from build123d import *

# Parameters (mm, degrees)
COMPACT_HORN_CENTER_OD6P9_PROFILE_R        = 3.45
COMPACT_HORN_CENTER_OD6P9_DEPTH            = 1.5
HORIZONTAL_BLADES_ASSUMED_WIDTH4_PROFILE_W = 16.3
HORIZONTAL_BLADES_ASSUMED_WIDTH4_PROFILE_H = 4
HORIZONTAL_BLADES_ASSUMED_WIDTH4_DEPTH     = 1.5
VERTICAL_BLADES_ASSUMED_WIDTH4_PROFILE_W   = 4
VERTICAL_BLADES_ASSUMED_WIDTH4_PROFILE_H   = 16.3
VERTICAL_BLADES_ASSUMED_WIDTH4_DEPTH       = 1.5
ROUNDED_BLADE_TIPS_R                       = 2
ROUNDED_TIPS_SPAN20P3_DEPTH                = 1.5
HUB_TOTAL_HEIGHT2P5_START                  = -1
HUB_TOTAL_HEIGHT2P5_PROFILE_R              = 3.45
HUB_TOTAL_HEIGHT2P5_DEPTH                  = 1
PURCHASED_SPLINE_INTERNALS_OMITTED_START   = -50
PURCHASED_SPLINE_INTERNALS_OMITTED_PROFI_R = 2.55
PURCHASED_SPLINE_INTERNALS_OMITTED_DEPTH   = 65.432428763
UNMODIFIED_STOCK_PILOT_HOLES_START         = -50
UNMODIFIED_STOCK_PILOT_HOLES_PROFILE_R     = 0.5
UNMODIFIED_STOCK_PILOT_HOLES_DEPTH         = 65.432428763


with BuildPart() as part:
    # Compact_horn_center_OD6p9_profile → Compact_horn_center_OD6p9 (new body)
    with BuildSketch(Plane.XY):
        Circle(COMPACT_HORN_CENTER_OD6P9_PROFILE_R)
    extrude(amount=COMPACT_HORN_CENTER_OD6P9_DEPTH)

    # Horizontal_blades_assumed_width4_profile → Horizontal_blades_assumed_width4 (add)
    with BuildSketch(Plane.XY):
        Rectangle(HORIZONTAL_BLADES_ASSUMED_WIDTH4_PROFILE_W, HORIZONTAL_BLADES_ASSUMED_WIDTH4_PROFILE_H)
    extrude(amount=HORIZONTAL_BLADES_ASSUMED_WIDTH4_DEPTH)

    # Vertical_blades_assumed_width4_profile → Vertical_blades_assumed_width4 (add)
    with BuildSketch(Plane.XY):
        Rectangle(VERTICAL_BLADES_ASSUMED_WIDTH4_PROFILE_W, VERTICAL_BLADES_ASSUMED_WIDTH4_PROFILE_H)
    extrude(amount=VERTICAL_BLADES_ASSUMED_WIDTH4_DEPTH)

    # Rounded_blade_tips → Rounded_tips_span20p3 (add)
    with BuildSketch(Plane.XY):
        with Locations((8.15, 0)):
            Circle(ROUNDED_BLADE_TIPS_R)
        with Locations((-8.15, 0)):
            Circle(ROUNDED_BLADE_TIPS_R)
        with Locations((0, 8.15)):
            Circle(ROUNDED_BLADE_TIPS_R)
        with Locations((0, -8.15)):
            Circle(ROUNDED_BLADE_TIPS_R)
    extrude(amount=ROUNDED_TIPS_SPAN20P3_DEPTH)

    # Hub_total_height2p5_profile → Hub_total_height2p5 (add)
    with BuildSketch(Plane.XY.offset(HUB_TOTAL_HEIGHT2P5_START)):
        with Locations(Location((0, 0, 0), (0, 0, 215.43015836))):
            Circle(HUB_TOTAL_HEIGHT2P5_PROFILE_R)
    extrude(amount=HUB_TOTAL_HEIGHT2P5_DEPTH)

    # Purchased_spline_internals_omitted_profile → Purchased_spline_internals_omitted (cut, through all)
    with BuildSketch(Plane.XY.offset(PURCHASED_SPLINE_INTERNALS_OMITTED_START)):
        Circle(PURCHASED_SPLINE_INTERNALS_OMITTED_PROFI_R)
    extrude(amount=PURCHASED_SPLINE_INTERNALS_OMITTED_DEPTH, mode=Mode.SUBTRACT)

    # Unmodified_stock_pilot_holes_profile → Unmodified_stock_pilot_holes (cut, through all)
    with BuildSketch(Plane.XY.offset(UNMODIFIED_STOCK_PILOT_HOLES_START)):
        with Locations((-8.3, 0)):
            Circle(UNMODIFIED_STOCK_PILOT_HOLES_PROFILE_R)
        with Locations((-6.3, 0)):
            Circle(UNMODIFIED_STOCK_PILOT_HOLES_PROFILE_R)
        with Locations((-4.3, 0)):
            Circle(UNMODIFIED_STOCK_PILOT_HOLES_PROFILE_R)
        with Locations((4.3, 0)):
            Circle(UNMODIFIED_STOCK_PILOT_HOLES_PROFILE_R)
        with Locations((6.3, 0)):
            Circle(UNMODIFIED_STOCK_PILOT_HOLES_PROFILE_R)
        with Locations((8.3, 0)):
            Circle(UNMODIFIED_STOCK_PILOT_HOLES_PROFILE_R)
        with Locations((0, -8.3)):
            Circle(UNMODIFIED_STOCK_PILOT_HOLES_PROFILE_R)
        with Locations((0, -6.3)):
            Circle(UNMODIFIED_STOCK_PILOT_HOLES_PROFILE_R)
        with Locations((0, -4.3)):
            Circle(UNMODIFIED_STOCK_PILOT_HOLES_PROFILE_R)
        with Locations((0, 4.3)):
            Circle(UNMODIFIED_STOCK_PILOT_HOLES_PROFILE_R)
        with Locations((0, 6.3)):
            Circle(UNMODIFIED_STOCK_PILOT_HOLES_PROFILE_R)
        with Locations((0, 8.3)):
            Circle(UNMODIFIED_STOCK_PILOT_HOLES_PROFILE_R)
    extrude(amount=UNMODIFIED_STOCK_PILOT_HOLES_DEPTH, mode=Mode.SUBTRACT)


solid = part.part
Input: part model. Units: mm. Frame: model coordinates. A direction names the side the tool comes from. Round coordinates to 2 decimals unless told otherwise and drop trailing zeros. Order: outer loops, then holes, each group sorted by start corner. A loop starts at its lowest first (then second) coordinate and runs counter-clockwise, first axis right, second up. Notation, with made-up numbers: (5.25, 48.25) - (29.25, 48.25) arc R23 ccw to (29.25, 83.25) - close; hole circle Ø3 at (3.25, -27). An arc over 180 degrees is marked (long way). Answer as a JSON object with one key per item and string values. Group by question number.
(1) Pin query (flat end, axial travel): P1, Ø2, axis at x = -6, y = 0.5, coming from the -Z side; P2, Ø1.2, axis at y = -6.5, z = 1, coming from the +X side; P3, Ø0.8, axis at x = 6, z = 0.5, coming from the -Y side. Return the tip coordinate at first contact, or that it passes through.
(2) Draft query along Y for faces 1 (the face through (-0.108, 3.812, 0.739)), 2 (the face through (-0.065, -5.804, 0.739)), 3 (the face through (2, -6, 1)), 4 (the face through (5, 2, 1)). Return one class per face: released by +Y, released by -Y, zero draft, split by the parting line, or undercut.
(3) Cut plane C-C (z = 0.8). Count the separate pieces of the cut face and the enclosed holes in it, then the cut area to 3 significant figures.
(4) Material intervals for probe 1 along Y at (x, z) = (8.3, 0.8); probe 2 along X at (y, z) = (-4.3, 0.6); probe 3 along X at (y, z) = (-3.75, 0.3), sorted ascending. Write a range as from..to.
(5) Reachability of faces 5 (the face through (-2, 2, 1.5)), 6 (the face through (2, 5, 1)), 7 (the face through (-6.8, 0, 0.7)), 8 (the face through (-2, 5, 1)), 9 (the face through (-2, -6, 1)) from +Z, -Z, +X, -X, +Y, -Y: full face, straight path, thin tool, end or side. Return the list, or none.
(6) Cut plane A-A (x = -4.3). Return loops of the section in (y, z), then the cut area to 3 significant figures.
(7) Cut plane D-D (z = -0.55). Return loops of the section in (x, y).
Here are the results:
{
 "1": {"P1": "stops at z = 0", "P2": "stops at x = 2", "P3": "stops at y = -2"},
 "2": {"face 1": "undercut", "face 2": "undercut", "face 3": "zero draft", "face 4": "released by +Y"},
 "3": {"separate pieces": "1", "enclosed holes": "13", "area": "111 mm^2"},
 "4": {"probe 1": "y = -1.99..-0.5, 0.5..1.99", "probe 2": "x = -2..-0.5, 0.5..2", "probe 3": "x = -2..2"},
 "5": {"face 5": "+Z, +X, -X, +Y, -Y", "face 6": "+Z, -Z, +X, +Y", "face 7": "+Z, -Z", "face 8": "+Z, -Z, -X, +Y", "face 9": "+Z, -Z, -X, -Y"},
 "6": {"outline": "(-2, 0) - (-0.5, 0) - (-0.5, 1.5) - (-2, 1.5) - close; (0.5, 0) - (2, 0) - (2, 1.5) - (0.5, 1.5) - close", "area": "4.50 mm^2"},
 "7": {"outline": "circle Ø6.9 at (0, 0); hole circle Ø5.1 at (0, 0)"}
}
